Can you work these out from the model? Positions are in its coordinate system, mm. A direction names the side the tool comes from. Give positions to 0.01 mm unless a question says otherwise; leave off trailing zeros. Order: outer loops, then holes, each group sorted by start corner. A loop starts at its lowest first (then second) coordinate and runs counter-clockwise, first axis right, second up. Notation, with made-up numbers: M 70,-26.75 L 122,-26.75 A24 ccw 122,8.25 Z; hole C -28,22 d5. An arc over 180 degrees is marked long. One line per question, with ' | ' between items. Start each with the question number.
1) If we section it at B-B, the plane z = 0: Please give me the cut outline in (x, y), plus the area to 3 significant figures.
2) Please list where these lines run through material, in increasing order: line 1 along Z through (x, y) = (216, 0); line 2 along Z through (x, y) = (-29, 0); line 3 along X through (y, z) = (16, -46.5). Write a range as [from, to].
3) If we section it at D-D, the plane x = 62.5: Please give me the cut outline in (y, z), plus the area to 3 significant figures.
4) I'm going to push flat-ended pins straight in: pin 1 Ø1.5 at (x, z) = (-79, 15) entering from +Y; pin 2 Ø5 at (y, z) = (-40.5, -39) entering from +X; pin 3 Ø5 at (x, y) = (118, 5) entering from +Z. Where does each tip first touch, or does it pass through?
5) If we section it at A-A, the plane x = 195.5: Please give me the cut outline in (y, z), plus the area to 3 significant figures.
6) For faces 1 (the flat face through (0, 0, 0)), 2 (the cylindrical face through (201.638, -2.606, 19.848)), 3 (the flat face through (-127.508, 19, -6)), which set-ups out of +Z, -Z, +X, -X, +Y, -Y let a thin tool reach every point of the face, with its end or its side?
7) Thinking about a two-plate mould opening in Z: for faces 4 (the flat face through (100.584, 0, 0)), 5 (the flat face through (100.584, 28, 1)), 6 (the cylindrical face through (-62.861, -26.377, 8.306)), 7 (the cylindrical face through (-62.86, 19.38, 0.85)), which applies, +Z half, -Z half, draft (parallel to the pull), parting line (faces both ways), or undercut?
```python
from build123d import *

# Parameters (mm, degrees)
F0_R     = 64.132843
F1_DEPTH = 100.584
F2_R     = 27.60981
F2_R_2   = 20.017869
F3_DEPTH = 204.978
F4_R     = 27.653728
F4_R_2   = 19.400153
F5_DEPTH = 127.508


with BuildPart() as f1:
    # F0 (on Right) → F1 (new body)
    with BuildSketch(Plane.YZ):
        Circle(F0_R)
    extrude(amount=F1_DEPTH)

    # F2 (on face) → F3 (join)
    with BuildSketch(Plane.YZ.offset(100.584)):
        Circle(F2_R)
        Circle(F2_R_2, mode=Mode.SUBTRACT)
    extrude(amount=F3_DEPTH)

    # F4 (on face) → F5 (join)
    with BuildSketch(Plane(origin=(0, 0, 0), x_dir=(0, -1, 0), z_dir=(-1, 0, 0))):
        Circle(F4_R)
        Circle(F4_R_2, mode=Mode.SUBTRACT)
    extrude(amount=F5_DEPTH)


solid = f1.part
```
Results found:
1) outline: M -127.51,-27.65 L 0,-27.65 L 0,-64.13 L 100.58,-64.13 L 100.58,-27.61 L 305.56,-27.61 L 305.56,-20.02 L 100.58,-20.02 L 100.58,20.02 L 305.56,20.02 L 305.56,27.61 L 100.58,27.61 L 100.58,64.13 L 0,64.13 L 0,27.65 L -127.51,27.65 L -127.51,19.4 L 0,19.4 L 0,-19.4 L -127.51,-19.4 Z | area: 18,100 mm²
2) line 1: z = [-27.61, -20.02], [20.02, 27.61] | line 2: z = [-27.65, -19.4], [19.4, 27.65] | line 3: x = [0, 100.58]
3) outline: C 0,0 d128.27 | area: 12,900 mm²
4) pin 1: stops at y = 23.7 | pin 2: stops at x = 100.58 | pin 3: stops at z = 27.5
5) outline: C 0,0 d55.22; hole C 0,0 d40.04 | area: 1,140 mm²
6) face 1: -X | face 2: +X | face 3: +Z, -Z, -X, +Y, -Y
7) face 4: undercut | face 5: draft | face 6: parting line | face 7: undercut
